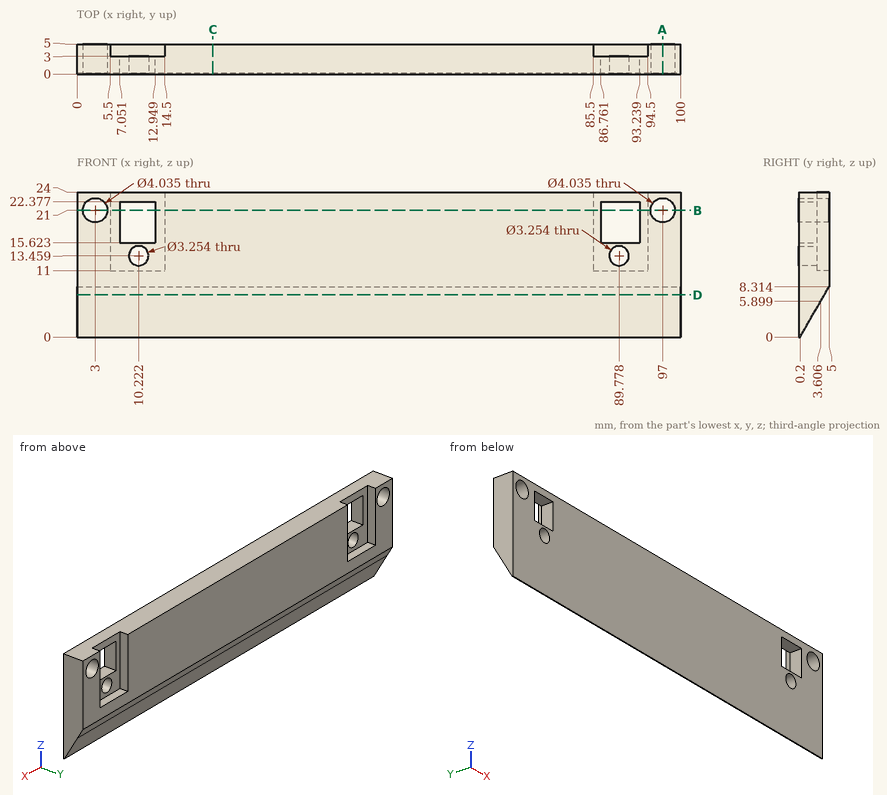
Here's the drawing with two shaded views (mm, measured from the low corner). I have some questions. Coordinates: 2 decimals unless noted, no trailing zeros. Order: outer loops, then holes, each group sorted by start corner. A loop starts at its lowest first (then second) coordinate and runs counter-clockwise, first axis right, second up. Notation, with made-up numbers: (17.25, -39.75) - (26.25, -39.75) arc R21 ccw to (26.25, -9.75) - close; hole circle Ø11 at (-3.75, 54). An arc over 180 degrees is marked (long way). Use CSV: the item, a comma, the result in double quotes. Start each with the question number.
1. I'm going to push flat-ended pins straight in: pin 1 (0.9 mm diameter, centred on y = 2, z = 20, fed in from -X); pin 2 (3 mm diameter, centred on x = 10.22, z = 13.46, fed in from +Y); pin 3 (1 mm diameter, centred on x = 55, y = 3.5, fed in from -Z); pin 4 (3 mm diameter, centred on x = 89.5, z = 4, fed in from +Y) (1 decimal). Where does each tip first touch, or does it pass through?
2. Suppose I cut it at D-D on z = 7. List the corners of the cut face in (x, y) for me.
3. Please list where these lines run through material, in increasing order: line 1 (X direction, y = 0.85, z = 17); line 2 (X direction, y = 2.9, z = 21); line 3 (X direction, y = 4.7, z = 21). Write a range as from..to.
4. Suppose I cut it at B-B on z = 21. List the corners of the cut face in (x, y) for me.
5. Suppose I cut it at A-A on x = 97. List the corners of the cut face in (y, z) for me.
6. Suppose I cut it at C-C on x = 22.5. List the corners of the cut face in (y, z) for me, then the cut area to 3 significant figures.
Output:
1,pin 1,"stops at x = 0"
1,pin 2,"passes through"
1,pin 3,"stops at z = 4.85"
1,pin 4,"stops at y = 3.4"
2,outline,"(0, 0) - (100, 0) - (100, 4.24) - (0, 4.24) - close"
3,line 1,"x = 0..7.05, 12.95..86.76, 93.24..100"
3,line 2,"x = 0..0.98, 5.02..7.05, 12.95..86.76, 93.24..94.98, 99.02..100"
3,line 3,"x = 0..0.98, 5.02..5.5, 14.5..85.5, 94.5..94.98, 99.02..100"
4,outline,"(0, 0) - (0.98, 0) - (0.98, 5) - (0, 5) - close; (5.02, 0) - (7.05, 0) - (7.05, 3) - (5.5, 3) - (5.5, 5) - (5.02, 5) - close; (12.95, 0) - (86.76, 0) - (86.76, 3) - (85.5, 3) - (85.5, 5) - (14.5, 5) - (14.5, 3) - (12.95, 3) - close; (93.24, 0) - (94.98, 0) - (94.98, 5) - (94.5, 5) - (94.5, 3) - (93.24, 3) - close; (99.02, 0) - (100, 0) - (100, 5) - (99.02, 5) - close"
5,outline,"(0, 0) - (0.2, 0) - (5, 8.31) - (5, 18.98) - (0, 18.98) - close; (0, 23.02) - (5, 23.02) - (5, 24) - (0, 24) - close"
6,outline,"(0, 0) - (0.2, 0) - (5, 8.31) - (5, 24) - (0, 24) - close"
6,area,"100 mm2"
